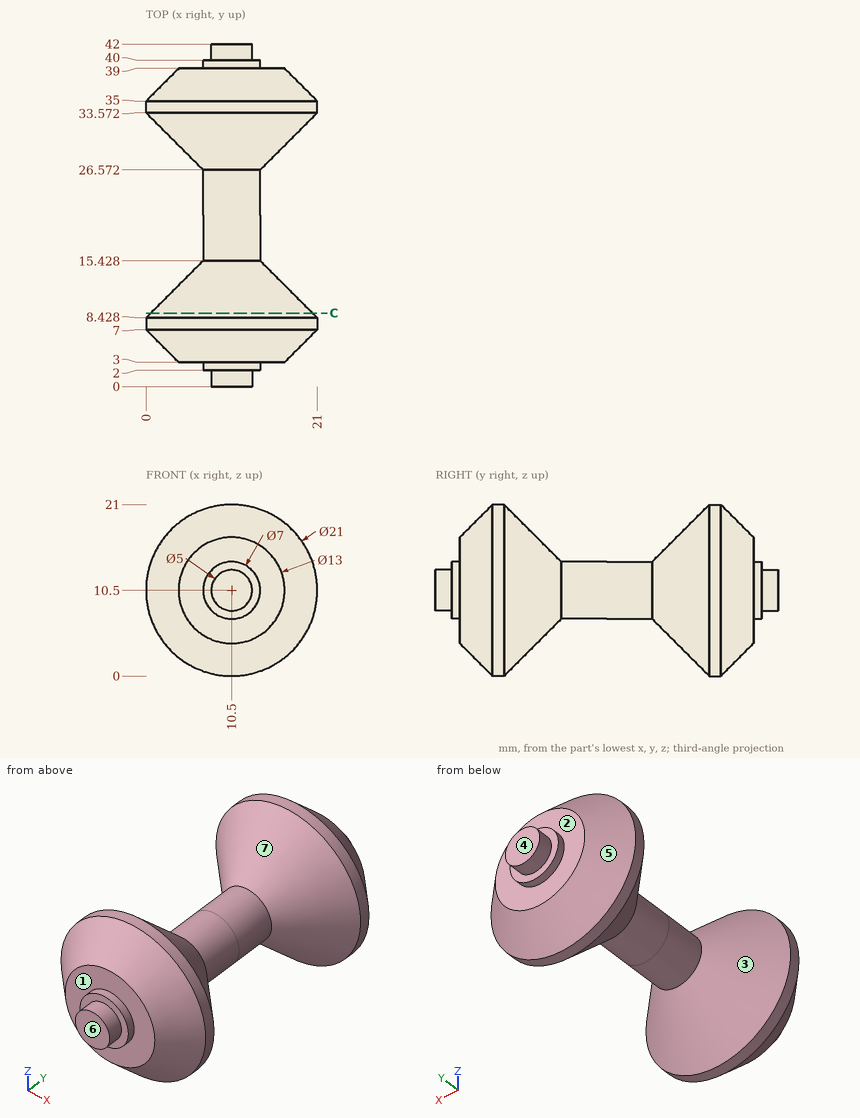
The drawing under review shows one solid part. Ordinate dimensions are in mm from its lowest x, y, z. A direction names the side the tool comes from. Round coordinates to 2 decimals unless told otherwise and drop trailing zeros. Write each loop counter-clockwise with the first axis right and the second up, starting at its lowest first coordinate (ties: lowest second). Pieces come first, ordered by that corner, then holes. Notation, with made-up numbers: (34.25, 82.5) - (86.25, 82.5) arc R26 cw to (86.25, 120.5) - close; hole circle Ø4 at (62, 5.5). An arc over 180 degrees is marked (long way). Write each question's results on one line, items separated by ' | '.
Item 1: For pin 1 (3 mm diameter, centred on x = 12, y = 18.5, fed in from -Z); pin 2 (5 mm diameter, centred on x = 9, z = 16, fed in from +Y); pin 3 (12 mm diameter, centred on x = 9, y = 21.5, fed in from -Z); pin 4 (8 mm diameter, centred on y = 32.5, z = 7.5, fed in from +X), all flat-tipped, find the tip position at first contact; note any pin that passes through.
Calculated:
pin 1: stops at z = 7 | pin 2: stops at y = 40 | pin 3: stops at z = 6.18 | pin 4: stops at x = 21
Item 2: Draft analysis for pull direction Y (two halves, no side actions). For the marked faces 5, 6 and 7, state which applies: pulls with the +Y half, pulls with the -Y half, needs draft (parallel to the pull), parting line crosses it, or undercut.
Calculated:
face 5: pulls with the +Y half | face 6: pulls with the -Y half | face 7: undercut
Item 3: To check wall thickness, follow line 1 along Y through (x, z) = (17.5, 13) (1 decimal); line 2 along Y through (x, z) = (16.5, 17.5); line 3 along Z through (x, y) = (18, 33) (1 decimal). State the ranges of each line that lie inside material, in increasing order. Write a range as from..to.
Calculated:
line 1: y = 3.9..11.5, 30.5..38.1 | line 2: y = 5.72..9.71, 32.29..36.28 | line 3: z = 4..17
Item 4: Take a section at C-C on y = 9. State the section outline as (x, z) points, then the cut area to 3 significant figures.
Calculated:
outline: circle Ø19.86 at (10.5, 10.5) | area: 310 mm^2
Item 5: For the marked faces 1, 2, 3 and 4, list the 3-axis set-ups (+Z, -Z, +X, -X, +Y, -Y) from which the entire face can be reached by the end or side of a thin tool; tool diameter is ignored.
Calculated:
face 1: -Y | face 2: +Y | face 3: none | face 4: +Z, -Z, +X, -X, +Y
